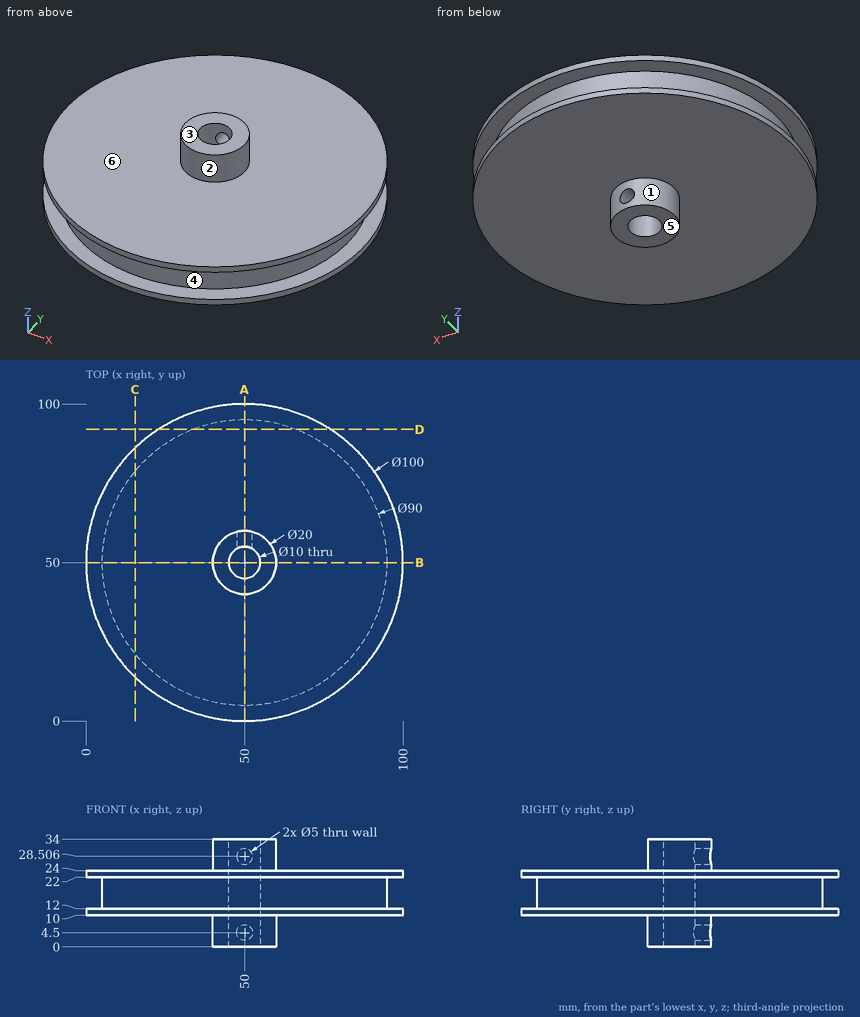
Answer from the drawing. Dimensions are ordinates in mm from the lowest x, y and z of the part. A direction names the side the tool comes from. Give positions to 0.01 mm unless a question says otherwise; leave off trailing zeros. Loops run counter-clockwise (first coordinate to the right, second up) from the corner with the lowest first, then second, coordinate; pieces in that order, holes last.
Item 1: The part is cut by section A-A (x = 50). Give the number of separate pieces and of enclosed holes in the cut face, and give its area (3 significant figures).
Item 2: For the marked faces 1, 2 and 3, determine the directions among +Z, -Z, +X, -X, +Y, -Y from which every point of the face is accessible in a straight line to the end or side of a thin tool.
Item 3: Find the intervals of material crossed by line 1 along Z through (x, y) = (50, 56); line 2 along Z through (x, y) = (38, 44.5); line 3 along Y through (x, z) = (50, 27), in increasing order.
Item 4: Each of these flat-tipped pins is pushed along its axis until it touches: pin 1 Ø3 at (x, z) = (68, 20) entering from -Y (1 decimal); pin 2 Ø8 at (x, y) = (19.5, 40.5) entering from -Z; pin 3 Ø8 at (x, y) = (50, 50) entering from +Z; pin 4 Ø6 at (x, z) = (50, 28.51) entering from +Y. Where does it stop, or does it pass through?
Item 5: The mould has two halves that part along Z. Classify the marked faces 4, 5 and 6: released by +Z, released by -Z, zero draft, split by the parting line, or undercut.
Item 6: The part is cut by section C-C (x = 15.5). Write down the section's boundary in (y, z).
Item 7: The part is cut by section D-D (y = 92). Write down the section's boundary in (x, z) (1 decimal), and give its area (3 significant figures).
Item 8: The part is cut by section B-B (y = 50). Write down the section's boundary in (x, z).
Taken from the geometry:
1. separate pieces: 4
1. enclosed holes: 0
1. area: 1,310 mm2
2. face 1: -Z
2. face 2: +Z
2. face 3: +Z, +X, -X, +Y, -Y
3. line 1: z = 0 to 2, 7 to 26.01, 31.01 to 34
3. line 2: z = 10 to 24
3. line 3: y = 40 to 45
4. pin 1: stops at y = 8.1
4. pin 2: stops at z = 10
4. pin 3: passes through
4. pin 4: stops at y = 60
5. face 4: undercut
5. face 5: released by -Z
5. face 6: released by +Z
6. outline: (13.81, 10) - (86.19, 10) - (86.19, 12) - (78.89, 12) - (78.89, 22) - (86.19, 22) - (86.19, 24) - (13.81, 24) - (13.81, 22) - (21.11, 22) - (21.11, 12) - (13.81, 12) - close
7. outline: (22.9, 10) - (77.1, 10) - (77.1, 12) - (66.2, 12) - (66.2, 22) - (77.1, 22) - (77.1, 24) - (22.9, 24) - (22.9, 22) - (33.8, 22) - (33.8, 12) - (22.9, 12) - close
7. area: 540 mm2
8. outline: (0, 10) - (40, 10) - (40, 0) - (45, 0) - (45, 34) - (40, 34) - (40, 24) - (0, 24) - (0, 22) - (5, 22) - (5, 12) - (0, 12) - close; (55, 0) - (60, 0) - (60, 10) - (100, 10) - (100, 12) - (95, 12) - (95, 22) - (100, 22) - (100, 24) - (60, 24) - (60, 34) - (55, 34) - close
